CAD build for the part. Positions are in the model's coordinates, mm. A direction names the side the tool comes from. Give positions to 0.01 mm unless a question says otherwise; leave off trailing zeros. Order: outer loops, then holes, each group sorted by start corner. A loop starts at its lowest first (then second) coordinate and runs counter-clockwise, first axis right, second up.
Item 1: Band-saw the part on B-B on y = 2.5. Count the separate pieces of the cut face and the enclosed holes in it, plus the area to 3 significant figures.
Item 2: Band-saw the part on A-A on x = 44.45. Give the cut face in (y, z), plus the area to 3 significant figures.
Item 3: Flat gauge pins, fed straight in: P1, Ø5, axis at x = 12.5, y = 3, coming from the +Z side; P2, Ø6, axis at x = -18, z = -12, coming from the +Y side; P3, Ø2, axis at y = 1.5, z = -21.5, coming from the -X side; P4, Ø5, axis at x = -21.5, y = 11.5, coming from the +Z side. Where does each tip first touch, or does it go through?
Item 4: Band-saw the part on C-C on z = -5. Give the cut face in (x, y), plus the area to 3 significant figures.
Item 5: Two-plate mould, pull along X, no slides. Class faces 3 (the cylindrical face through (42.42, 6.26, -35.78)), 4 (the cylindrical face through (-42.42, 6.26, -37.88)), 5 (the cylindrical face through (49.351, 6.439, -40.382)), 6 (the flat face through (-39, 6, -31.75)): released by +X, released by -X, zero draft, split by the parting line, or undercut.
Item 6: Band-saw the part on D-D on z = -10. Give the cut face in (x, y), plus the area to 3 significant figures.
Item 7: Wall check: L1, parallel to X at y = 7, z = -36.83; L2, parallel to X at y = 11.5, z = -35; L3, parallel to Z at x = 46, y = 4. Give the ranges that are in metal, low to high.
Item 8: Which spindle directions (+Z, -Z, +X, -X, +Y, -Y) get a long thin tool onto all of the face, cutting with end or side? Do faces 1 (the cylindrical face through (-49.351, 6.439, -40.382)), 2 (the flat face through (39, 6, -31.75)). Say none if no direction does.
```python
from build123d import *

# Parameters (mm, degrees)
SKETCH2_R           = 2.286
BOSS_EXTRUDE2_DEPTH = 12.7
FILLET1_R           = 5.08
FILLET2_R           = 12.7


# Some blends are built 0.0001 mm under size
with BuildPart() as part:
    # Sketch2 → Boss-Extrude2 (new body)
    with BuildSketch(Plane(origin=(0, 0, 0), x_dir=(1, 0, 0), z_dir=(0, 1, 0))):
        Polygon((-6.35, 0), (6.35, 0), (25.4, 31.75), (50.8, 31.75), (50.8, 41.91), (-50.8, 41.91), (-50.8, 31.75), (-25.4, 31.75), align=None)
        with Locations(Location((0, 19.05, 0), (0, 0, 270))):
            Circle(SKETCH2_R, mode=Mode.SUBTRACT)
        with Locations(Location((0, 6.35, 0), (0, 0, 270))):
            Circle(SKETCH2_R, mode=Mode.SUBTRACT)
        with Locations(Location((44.45, 36.83, 0), (0, 0, 270))):
            Circle(SKETCH2_R, mode=Mode.SUBTRACT)
        with Locations(Location((-44.45, 36.83, 0), (0, 0, 90))):
            Circle(SKETCH2_R, mode=Mode.SUBTRACT)
    extrude(amount=BOSS_EXTRUDE2_DEPTH)

    # Fillet1
    fillet1_edges = [part.edges().sort_by_distance(p)[0] for p in [
        (50.8, 6.35, -41.91),
        (50.8, 6.35, -31.75),
        (-50.8, 6.35, -41.91),
        (-50.8, 6.35, -31.75),
    ]]
    fillet(fillet1_edges, radius=FILLET1_R - 0.0001)  # a hair under: the kernel refuses the full size

    # Fillet2
    # the kernel refuses this fillet: 12.7 mm, written as the material it adds along each edge
    with BuildSketch(Plane(origin=(-25.4, 0, -31.75), x_dir=(0.5144957554275261, 0, 0.8574929257125444), z_dir=(0, 1, 0)), Plane(origin=(25.4, 0, -31.75), x_dir=(1, 0, 0), z_dir=(0, 1, 0))) as fillet2_piece_1:
        with BuildLine():
            CenterArc((FILLET2_R * 0.566190378969, -FILLET2_R), FILLET2_R, 90, 59.036243468)
            Line((-FILLET2_R * 0.291302546743, -FILLET2_R * 0.485504244572), (0, 0))
            Line((0, 0), (FILLET2_R * 0.566190378969, 0))
        make_face()
    extrude(amount=12.7)
    # the kernel refuses this fillet: 12.7 mm, written as the material it takes off along each edge
    with BuildSketch(Plane(origin=(-6.35, -17.976544532, 0), x_dir=(1, 0, 0), z_dir=(0, 1, 0)), Plane(origin=(6.35, -17.976544532, 0), x_dir=(0.514495755427526, 0, -0.8574929257125444), z_dir=(0, 1, 0))) as fillet2_2_piece_1:
        with BuildLine():
            CenterArc((FILLET2_R * 0.566190378969, FILLET2_R), FILLET2_R, 210.963756532, 59.036243468)
            Line((-FILLET2_R * 0.291302546743, FILLET2_R * 0.485504244572), (0, 0))
            Line((0, 0), (FILLET2_R * 0.566190378969, 0))
        make_face()
    extrude(amount=48.653089065, mode=Mode.SUBTRACT)


solid = part.part
```
The answers:
1. separate pieces: 1
1. enclosed holes: 4
1. area: 1,950 mm2
2. outline: (0, -41.91) - (12.7, -41.91) - (12.7, -39.12) - (0, -39.12) - close; (0, -34.54) - (12.7, -34.54) - (12.7, -31.75) - (0, -31.75) - close
2. area: 71.0 mm2
3. P1: stops at z = -6.08
3. P2: passes through
3. P3: stops at x = -19.85
3. P4: stops at z = -21.08
4. outline: (-9.26, 0) - (-1.84, 0) - (-1.84, 12.7) - (-9.26, 12.7) - close; (1.84, 0) - (9.26, 0) - (9.26, 12.7) - (1.84, 12.7) - close
4. area: 188 mm2
5. face 3: undercut
5. face 4: undercut
5. face 5: released by +X
5. face 6: zero draft
6. outline: (-12.35, 0) - (12.35, 0) - (12.35, 12.7) - (-12.35, 12.7) - close
6. area: 314 mm2
7. L1: x = -50.8 to -46.74, -42.16 to 42.16, 46.74 to 50.8
7. L2: x = -50.46 to -45.82, -43.08 to 43.08, 45.82 to 50.46
7. L3: z = -41.9 to -38.51, -35.15 to -31.76
8. face 1: -Z, -X, +Y, -Y
8. face 2: +Z, +X, +Y, -Y
